Can you work these out from the model? Positions are in its coordinate system, mm. Face numbers are marked on the shaded views. A direction names the side the tool comes from. Give positions to 0.01 mm unless a question says otherwise; leave off trailing zeros. Order: outer loops, then holes, each group sorted by start corner. A loop starts at its lowest first (then second) coordinate and runs counter-clockwise, first axis right, second up. Notation, with made-up numbers: (-34, 86) -> (11, 86) arc R4 cw to (11, 93) -> close; hole circle Ø5 at (20.5, 10). An arc over 180 degrees is marked (long way). Answer as CSV lines item,"result".
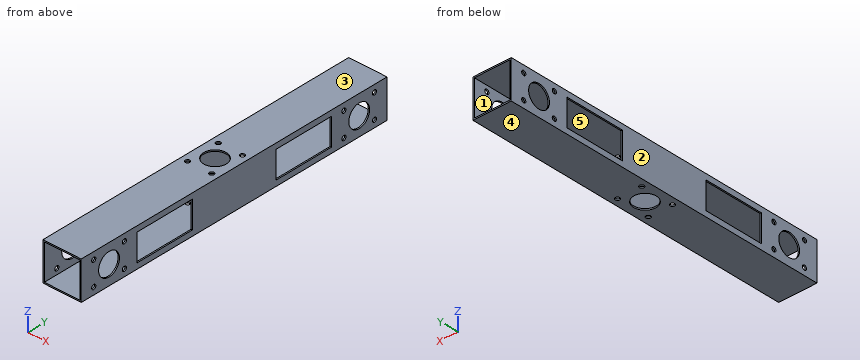
```python
from build123d import *

# Parameters (mm, degrees)
SKETCH1_W           = 25.4
SKETCH1_H           = 25.4
SKETCH1_W_2         = 23.6
SKETCH1_H_2         = 23.6
BOSS_EXTRUDE1_DEPTH = 220
SKETCH2_R           = 7.5
CUT_EXTRUDE1_DEPTH  = 25.4
SKETCH3_R           = 7.5
SKETCH3_W           = 18
SKETCH3_H           = 40
CUT_EXTRUDE2_DEPTH  = 25.4
SKETCH5_R           = 1.5
CUT_EXTRUDE4_DEPTH  = 25.4
SKETCH4_R           = 1.5
CUT_EXTRUDE5_DEPTH  = 25.4


with BuildPart() as part:
    # Sketch1 → Boss-Extrude1 (new body)
    with BuildSketch(Plane(origin=(0, 0, 0), x_dir=(1, 0, 0), z_dir=(0, 1, 0))):
        Rectangle(SKETCH1_W, SKETCH1_H)
        Rectangle(SKETCH1_W_2, SKETCH1_H_2, mode=Mode.SUBTRACT)
    extrude(amount=BOSS_EXTRUDE1_DEPTH)

    # Sketch2 → Cut-Extrude1 (cut)
    with BuildSketch(Plane(origin=(0, 0, -12.7), x_dir=(-1, 0, 0), z_dir=(0, 0, -1))):
        with Locations((0, 110)):
            Circle(SKETCH2_R)
    extrude(amount=-CUT_EXTRUDE1_DEPTH, mode=Mode.SUBTRACT)

    # Sketch3 → Cut-Extrude2 (cut)
    with BuildSketch(Plane(origin=(12.7, 0, 0), x_dir=(0, 0, -1), z_dir=(1, 0, 0))):
        with Locations((0, 20)):
            Circle(SKETCH3_R)
        with Locations(Location((0.307032613, 200, 0), (0, 0, 180))):
            Circle(SKETCH3_R)
        with Locations((0, 60)):
            Rectangle(SKETCH3_W, SKETCH3_H)
        with Locations((0, 160)):
            Rectangle(SKETCH3_W, SKETCH3_H)
    extrude(amount=-CUT_EXTRUDE2_DEPTH, mode=Mode.SUBTRACT)

    # Sketch5 → Cut-Extrude4 (cut)
    with BuildSketch(Plane(origin=(0, 0, -12.7), x_dir=(-1, 0, 0), z_dir=(0, 0, -1))):
        with Locations((8, 99)):
            Circle(SKETCH5_R)
        with Locations((8, 121)):
            Circle(SKETCH5_R)
        with Locations((-8, 121)):
            Circle(SKETCH5_R)
        with Locations((-8, 99)):
            Circle(SKETCH5_R)
    extrude(amount=-CUT_EXTRUDE4_DEPTH, mode=Mode.SUBTRACT)

    # Sketch4 → Cut-Extrude5 (cut)
    with BuildSketch(Plane.ZY.offset(12.7)):
        with Locations((8, 9)):
            Circle(SKETCH4_R)
        with Locations((8, 31)):
            Circle(SKETCH4_R)
        with Locations((-8, 9)):
            Circle(SKETCH4_R)
        with Locations((-8, 31)):
            Circle(SKETCH4_R)
        with Locations((8, 211)):
            Circle(SKETCH4_R)
        with Locations((-8, 211)):
            Circle(SKETCH4_R)
        with Locations((8, 189)):
            Circle(SKETCH4_R)
        with Locations((-8, 189)):
            Circle(SKETCH4_R)
    extrude(amount=-CUT_EXTRUDE5_DEPTH, mode=Mode.SUBTRACT)


solid = part.part
```
Item 1: Please list where these lines run through material, in increasing order: line 1 along Y through (x, z) = (12.55, 0); line 2 along Y through (x, z) = (8, -12.3); line 3 along Z through (x, y) = (-12.05, 189).
Numbers:
line 1,"y = 0 to 12.5, 27.5 to 40, 80 to 140, 180 to 192.51, 207.49 to 220"
line 2,"y = 0 to 97.5, 100.5 to 119.5, 122.5 to 220"
line 3,"z = -12.7 to -9.5, -6.5 to 6.5, 9.5 to 12.7"
Item 2: Imagine slicing it at D-D, the plane z = 0. Give the number of separate pieces and of enclosed holes in the cut face, then the cut area to 3 significant figures.
Numbers:
separate pieces,"10"
enclosed holes,"0"
area,"198 mm²"
Item 3: For the marked faces 4 and 5, which set-ups out of +Z, -Z, +X, -X, +Y, -Y let a thin tool reach every point of the face, with its end or its side?
Numbers:
face 4,"-Z, +X, -X, +Y, -Y"
face 5,"+Y, -Y"
Item 4: For pin 1 (2.5 mm diameter, centred on x = -8, y = 99, fed in from +Z), with a flat end and sliding along its axis, tell me the tip position at first contact or that it passes through.
Numbers:
pin 1,"passes through"
Item 5: Imagine slicing it at B-B, the plane y = 200. Please give me the cut outline in (x, z), then the cut area to 3 significant figures.
Numbers:
outline,"(-12.7, -12.7) -> (12.7, -12.7) -> (12.7, -7.81) -> (11.8, -7.81) -> (11.8, -11.8) -> (-11.8, -11.8) -> (-11.8, -7.81) -> (-12.7, -7.81) -> close; (-12.7, 7.19) -> (-11.8, 7.19) -> (-11.8, 11.8) -> (11.8, 11.8) -> (11.8, 7.19) -> (12.7, 7.19) -> (12.7, 12.7) -> (-12.7, 12.7) -> close"
area,"61.2 mm²"
Item 6: Imagine slicing it at C-C, the plane y = 150. Please give me the cut outline in (x, z).
Numbers:
outline,"(-12.7, -12.7) -> (12.7, -12.7) -> (12.7, -9) -> (11.8, -9) -> (11.8, -11.8) -> (-11.8, -11.8) -> (-11.8, -9) -> (-12.7, -9) -> close; (-12.7, 9) -> (-11.8, 9) -> (-11.8, 11.8) -> (11.8, 11.8) -> (11.8, 9) -> (12.7, 9) -> (12.7, 12.7) -> (-12.7, 12.7) -> close"
Item 7: Imagine slicing it at A-A, the plane y = 34.5. Please give me the cut outline in (x, z), then the cut area to 3 significant figures.
Numbers:
outline,"(-12.7, -12.7) -> (12.7, -12.7) -> (12.7, 12.7) -> (-12.7, 12.7) -> close; hole (-11.8, -11.8) -> (11.8, -11.8) -> (11.8, 11.8) -> (-11.8, 11.8) -> close"
area,"88.2 mm²"
Item 8: We'd pull the mould along Z, two halves only. Please class the marked faces 1, 2 and 3: released by +Z, released by -Z, zero draft, split by the parting line, or undercut.
Numbers:
face 1,"undercut"
face 2,"zero draft"
face 3,"released by +Z"
